from build123d import *

# Parameters (mm, degrees)
AUFSATZ_LINEAR_AUSTRAGEN1_DEPTH      = 242.5
SCHNITT_LINEAR_AUSTRAGEN1_DEPTH      = 255.22676885017438
SCHNITT_LINEAR_AUSTRAGEN1_DEPTH_BACK = 255.22676885017438
SKIZZE2_R                            = 40


with BuildPart() as part:
    # Skizze1 → Aufsatz-Linear austragen1 (new body)
    with BuildSketch(Plane(origin=(0, 0, 0), x_dir=(1, 0, 0), z_dir=(0, 1, 0))):
        with BuildLine():
            Line((-27.399999999999988, -65), (27.400000000000016, -65.00000000000001))
            ThreePointArc((27.400000000000016, -65.00000000000001), (36.30954544295052, -61.30954544295051), (40.00000000000002, -52.400000000000006))
            Line((40.00000000000002, -52.400000000000006), (40, 52.400000000000006))
            ThreePointArc((40, 52.400000000000006), (36.309545442950494, 61.30954544295051), (27.4, 65))
            Line((27.4, 65), (-27.399999999999995, 64.99999999999997))
            ThreePointArc((-27.399999999999995, 64.99999999999997), (-36.30954544295047, 61.30954544295047), (-39.99999999999999, 52.39999999999999))
            Line((-39.99999999999999, 52.39999999999999), (-39.999999999999986, -52.400000000000006))
            ThreePointArc((-39.999999999999986, -52.400000000000006), (-36.30954544295049, -61.3095454429505), (-27.399999999999988, -65))
        make_face()
        with BuildLine():
            Line((-27.39999999999999, -58.7), (27.400000000000016, -58.7))
            ThreePointArc((27.400000000000016, -58.7), (31.854772721475264, -56.85477272147525), (33.70000000000002, -52.400000000000006))
            Line((33.70000000000002, -52.400000000000006), (33.7, 52.400000000000006))
            ThreePointArc((33.7, 52.400000000000006), (31.854772721475253, 56.85477272147526), (27.400000000000002, 58.7))
            Line((27.400000000000002, 58.7), (-27.39999999999999, 58.7))
            ThreePointArc((-27.39999999999999, 58.7), (-31.854772721475243, 56.85477272147526), (-33.69999999999999, 52.400000000000006))
            Line((-33.69999999999999, 52.400000000000006), (-33.69999999999999, -52.400000000000006))
            ThreePointArc((-33.69999999999999, -52.400000000000006), (-31.85477272147524, -56.85477272147525), (-27.39999999999999, -58.7))
        make_face(mode=Mode.SUBTRACT)
    extrude(amount=AUFSATZ_LINEAR_AUSTRAGEN1_DEPTH)

    # Skizze2 → Schnitt-Linear austragen1 (cut, two sides: drawn at the far end of the back side and taken through both)
    with BuildSketch(Plane.XY.offset(-SCHNITT_LINEAR_AUSTRAGEN1_DEPTH_BACK)):
        Circle(SKIZZE2_R)
    extrude(amount=SCHNITT_LINEAR_AUSTRAGEN1_DEPTH + SCHNITT_LINEAR_AUSTRAGEN1_DEPTH_BACK, mode=Mode.SUBTRACT)


solid = part.part
Model file for the job. Use its own axes, mm. A direction names the side the tool comes from. Round coordinates to 2 decimals unless told otherwise and drop trailing zeros. Order: outer loops, then holes, each group sorted by start corner. A loop starts at its lowest first (then second) coordinate and runs counter-clockwise, first axis right, second up. Notation, with made-up numbers: M 4,83 L 11,83 A37 cw 11,121 Z; hole C 58,16 d2. An arc over 180 degrees is marked long. Write each question's results on one line, items separated by ' | '. Start each with the question number.
(1) Two-plate mould, pull along Z, no slides. Class faces 3 (the face through (-31.9, 130.48, 56.81)), 4 (the face through (-36.21, 119.55, -61.41)), 5 (the face through (-40, 120, -1)), 6 (the face through (-36.41, 119.55, 61.21)): pulls with the +Z half, pulls with the -Z half, needs draft (parallel to the pull), parting line crosses it, or undercut.
(2) Saw through at C-C, the plane z = 6.5. Give the cut face in (x, y), then the cut area to 3 significant figures.
(3) Drop a flat-ended pin along its axis: pin 1 (10 mm diameter, centred on x = -31, z = 25.5, fed in from -Y). Give the stop position or say it passes through.
(4) Saw through at A-A, the plane y = 196. Give the cut face in (x, z).
(5) Saw through at B-B, the plane x = 0. Give the cut face in (y, z), then the cut area to 3 significant figures.
(6) Probe probe 1 along Z at (x, y) = (13.5, 165.5); probe 2 along X at (y, z) = (171, 31); probe 3 along X at (y, z) = (93, -54). List the from-to ranges inside material, lowest first. Write a range as from..to.
(7) Which spindle directions (+Z, -Z, +X, -X, +Y, -Y) get a long thin tool onto all of the face, cutting with end or side? Do faces 1 (the face through (-36, 242.5, 0)), 2 (the face through (0, 134, -58.7)). Say none if no direction does.
Established:
1) face 3: undercut | face 4: pulls with the -Z half | face 5: needs draft | face 6: pulls with the +Z half
2) outline: M -40,0 A40 cw -33.7,21.55 L -33.7,242.5 L -40,242.5 Z; M 33.7,21.55 A40 cw 40,0 L 40,242.5 L 33.7,242.5 Z | area: 2,870 mm^2
3) pin 1: stops at y = 17.44
4) outline: M -40,-52.4 A12.6 ccw -27.4,-65 L 27.4,-65 A12.6 ccw 40,-52.4 L 40,52.4 A12.6 ccw 27.4,65 L -27.4,65 A12.6 ccw -40,52.4 Z; hole M -33.7,-52.4 A6.3 ccw -27.4,-58.7 L 27.4,-58.7 A6.3 ccw 33.7,-52.4 L 33.7,52.4 A6.3 ccw 27.4,58.7 L -27.4,58.7 A6.3 ccw -33.7,52.4 Z
5) outline: M 40,-65 L 242.5,-65 L 242.5,-58.7 L 40,-58.7 Z; M 40,58.7 L 242.5,58.7 L 242.5,65 L 40,65 Z | area: 2,550 mm^2
6) probe 1: z = -65..-58.7, 58.7..65 | probe 2: x = -40..-33.7, 33.7..40 | probe 3: x = -39.9..-33.49, 33.49..39.9
7) face 1: +Z, -Z, +X, -X, +Y | face 2: +Y, -Y
